Job drawing, mm, ordinate dimensions from the low corner. One solid piece. Give positions to 0.01 mm unless a question says otherwise; leave off trailing zeros. Loops run counter-clockwise (first coordinate to the right, second up) from the corner with the lowest first, then second, coordinate; pieces in that order, holes last. Notation, with made-up numbers: (65.25, 48) - (91.25, 48) arc R18 ccw to (91.25, 60) - close; hole circle Ø10 at (27, -24.75). An arc over 180 degrees is marked (long way). Use a Markdown table: item, result.
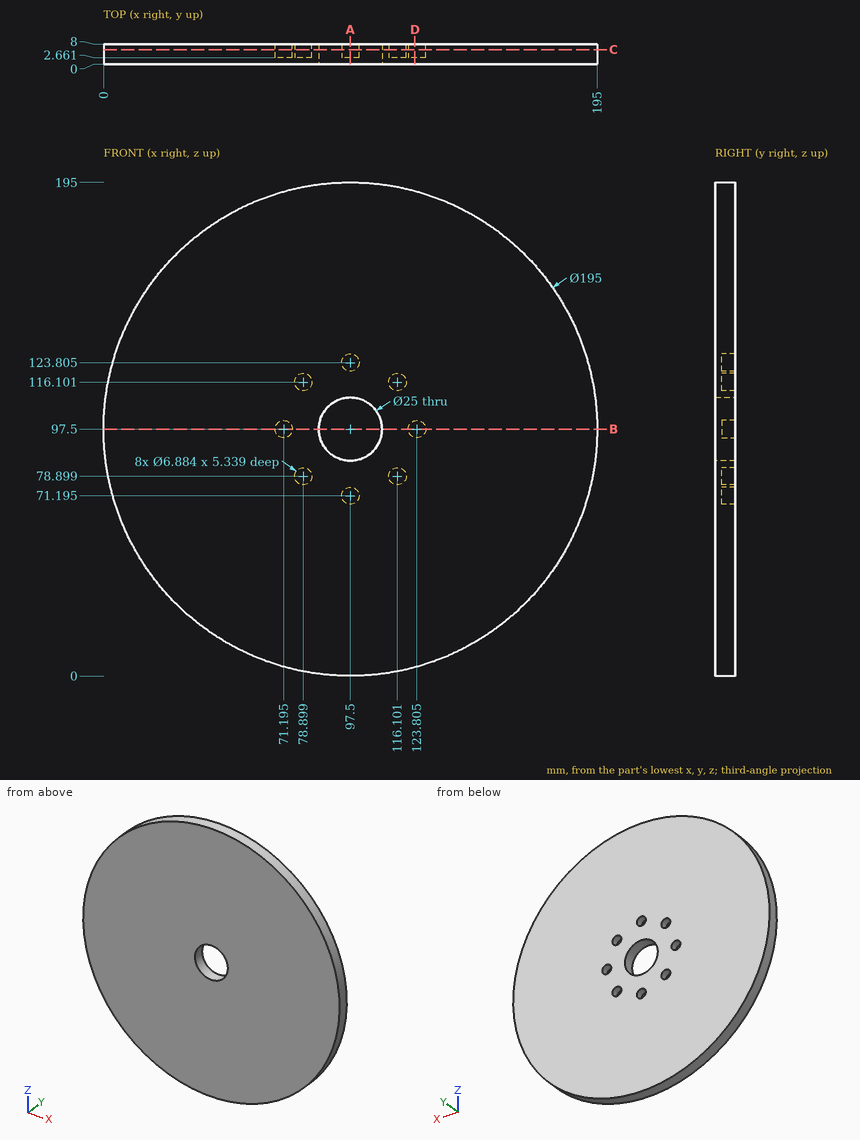
(1) Drill centre lines: probe 1 along X at (y, z) = (3.75, 97.5); probe 2 along X at (y, z) = (1.5, 97.5); probe 3 along Z at (x, y) = (118.5, 6.25) (1 decimal). Where is each one in solid material? Low to high. Write a range as [from, to].
Computed:
| item | result |
|---|---|
| probe 1 | [0, 67.75], [74.64, 85], [110, 120.36], [127.25, 195] |
| probe 2 | [0, 85], [110, 195] |
| probe 3 | [2.3, 76.4], [81.4, 113.6], [118.6, 192.7] |
(2) Slice it at B-B, the plane z = 97.5. Write the cut outline in (x, y), plus the area to 3 significant figures.
Computed:
| item | result |
|---|---|
| outline | (0, 0) - (85, 0) - (85, 8) - (74.64, 8) - (74.64, 2.66) - (67.75, 2.66) - (67.75, 8) - (0, 8) - close; (110, 0) - (195, 0) - (195, 8) - (127.25, 8) - (127.25, 2.66) - (120.36, 2.66) - (120.36, 8) - (110, 8) - close |
| area | 1,290 mm² |
(3) Slice it at D-D, the plane x = 123. Write the cut outline in (y, z).
Computed:
| item | result |
|---|---|
| outline | (0, 3.39) - (8, 3.39) - (8, 94.15) - (2.66, 94.15) - (2.66, 100.85) - (8, 100.85) - (8, 191.61) - (0, 191.61) - close |
(4) Slice it at C-C, the plane y = 5.75. Count the separate pieces of the cut face and the enclosed holes in it, plus the area to 3 significant figures.
Computed:
| item | result |
|---|---|
| separate pieces | 1 |
| enclosed holes | 9 |
| area | 29,100 mm² |
(5) Pin check, flat tips, straight feed: P1, Ø1.5, axis at x = 131, y = 1.5, coming from the +Z side (1 decimal); P2, Ø4, axis at x = 71.19, z = 97.5, coming from the +Y side. Stop position of each tip, or through.
Computed:
| item | result |
|---|---|
| P1 | z = 189.3 |
| P2 | y = 2.66 |
(6) Slice it at A-A, the plane x = 97.5. Write the cut outline in (y, z).
Computed:
| item | result |
|---|---|
| outline | (0, 0) - (8, 0) - (8, 67.75) - (2.66, 67.75) - (2.66, 74.64) - (8, 74.64) - (8, 85) - (0, 85) - close; (0, 110) - (8, 110) - (8, 120.36) - (2.66, 120.36) - (2.66, 127.25) - (8, 127.25) - (8, 195) - (0, 195) - close |
